Here's how the part is built. I have some questions about the finished solid (model axes, mm). Give positions to 0.01 mm unless a question says otherwise; leave off trailing zeros. Write each loop counter-clockwise with the first axis right and the second up, starting at its lowest first coordinate (ties: lowest second). Pieces come first, ordered by that corner, then holes. Notation, with made-up numbers: (13.5, -29.5) - (51.5, -29.5) arc R16 cw to (51.5, -4.5) - close; hole circle Ø11 at (84, 72). An arc over 180 degrees is marked (long way). Write each question's results on one line, items separated by ' | '. Start each with the question number.
Item 1: Please list where this line runs through material, in increasing order: line 1 along Y through (x, z) = (435, 2.8).
Item 2: Will these pins go through, and if not, where does the flat tip stop? P1, Ø1, axis at y = 1.5, z = 1.5, coming from the -X side; P2, Ø1.6, axis at y = 127.5, z = 1.5, coming from the +X side; P3, Ø1.6, axis at x = 429.5, z = 2.5, coming from the -Y side.
Item 3: Suppose I cut it at B-B on z = 1.15. Count the separate pieces of the cut face and the enclosed holes in it, then the cut area to 3 significant figures.
Item 4: Suppose I cut it at A-A on x = 299.5. List the corners of the cut face in (y, z) for me (1 decimal).
```python
from build123d import *

# Parameters (mm, degrees)
SKETCH1_W           = 71.428571428
SKETCH1_H           = 3.175
SKETCH1_W_2         = 71.428571429
BOSS_EXTRUDE1_DEPTH = 3.175


with BuildPart() as part:
    # Sketch1 → Boss-Extrude1 (new body)
    with BuildSketch(Plane.XY):
        Polygon((50.899754495, -0.012509515), (122.328325923, -0.012509515), (122.328325923, 3.162490485), (193.756897352, 3.162490485), (193.756897352, -0.012509515), (265.185468781, -0.012509515), (265.185468781, 3.162490485), (336.614040209, 3.162490485), (336.614040209, -0.012509515), (408.042611638, -0.012509515), (408.042611638, 3.162490485), (479.471183066, 3.162490485), (479.471183066, 126.337490485), (408.042611638, 126.337490485), (408.042611638, 129.512490485), (479.471183066, 129.512490485), (479.471183066, 252.687490485), (408.042611638, 252.687490485), (408.042611638, 255.862490485), (479.471183066, 255.862490485), (479.471183066, 294.037490485), (166.471183066, 294.037490485), (-20.528816934, 294.037490485), (-20.528816934, 255.862490485), (50.899754495, 255.862490485), (50.899754495, 252.687490485), (-20.528816934, 252.687490485), (-20.528816934, 129.512490485), (50.899754495, 129.512490485), (50.899754495, 126.337490485), (-20.528816934, 126.337490485), (-20.528816934, 3.162490485), (50.899754495, 3.162490485), align=None)
        with Locations((300.899754495, 127.924990485)):
            Rectangle(SKETCH1_W, SKETCH1_H, mode=Mode.SUBTRACT)
        with Locations((300.899754495, 254.274990485)):
            Rectangle(SKETCH1_W, SKETCH1_H, mode=Mode.SUBTRACT)
        with Locations((158.042611638, 127.924990485)):
            Rectangle(SKETCH1_W_2, SKETCH1_H, mode=Mode.SUBTRACT)
        with Locations((158.042611638, 254.274990485)):
            Rectangle(SKETCH1_W_2, SKETCH1_H, mode=Mode.SUBTRACT)
    extrude(amount=BOSS_EXTRUDE1_DEPTH)


solid = part.part
```
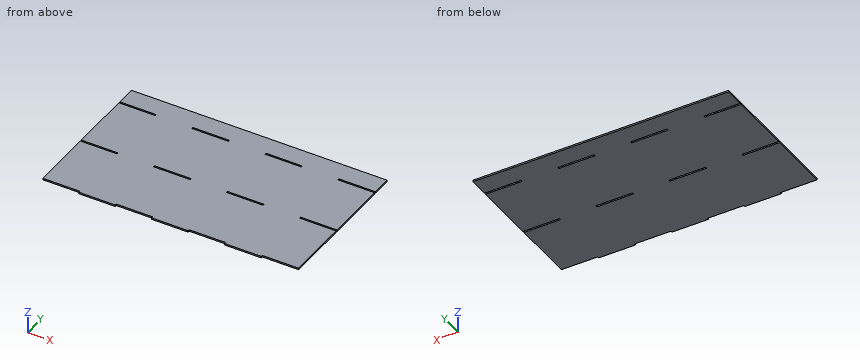
Checked values:
1) line 1: y = 3.16 to 126.34, 129.51 to 252.69, 255.86 to 294.04
2) P1: stops at x = 50.9 | P2: stops at x = 408.04 | P3: stops at y = 3.16
3) separate pieces: 1 | enclosed holes: 4 | area: 144,000 mm^2
4) outline: (3.2, 0) - (126.3, 0) - (126.3, 3.2) - (3.2, 3.2) - close; (129.5, 0) - (252.7, 0) - (252.7, 3.2) - (129.5, 3.2) - close; (255.9, 0) - (294, 0) - (294, 3.2) - (255.9, 3.2) - close
